from build123d import *

# Parameters (mm, degrees)
F1_W         = 50
F1_H         = 100
F2_DEPTH     = 30
F4_W         = 40
F4_H         = 90
F5_DEPTH     = 28
F6_SIZE      = 5
F7_T1_DEPTH  = 115
F7_T3_DEPTH  = 65
F8_W         = 40
F8_H         = 20
F9_DEPTH     = 40
F10_R        = 15.7450666382
F11_DEPTH    = 40
F12_R        = 5
F13_T1_DEPTH = 6.3508529611
F13_T3_DEPTH = 6.3508529611
F13_T5_DEPTH = 40.7168298797
F13_T7_DEPTH = 65.7168298797
F13_T9_DEPTH = 52.8584149398


# Not quite as in the source:
# - a fillet or chamfer that OpenCascade refuses, or shapes differently, is made with other operations: its cross-section is extruded or revolved along the edge and cut away or added


with BuildPart() as f2:
    # F1 (on face) → F2 (new body)
    with BuildSketch(Plane.XZ):
        Rectangle(F1_W, F1_H)
    extrude(amount=F2_DEPTH)

    # F4 (on face) → F5 (cut)
    with BuildSketch(Plane.XZ.offset(30)):
        with Locations((-0.4633623362, -0.2909506857)):
            Rectangle(F4_W, F4_H)
    extrude(amount=-F5_DEPTH, mode=Mode.SUBTRACT)

    # F6
    f6_edges = [f2.edges().sort_by_distance(p)[0] for p in [
        (25, -15, 50),
        (-25, -15, 50),
        (-25, -15, -50),
        (25, -15, -50),
    ]]
    chamfer(f6_edges, length=F6_SIZE)

    # F7: fillet of radius 5 on 4 edges, made by hand

    # F7_s2 → F7_t1 (cut)
    with BuildSketch(Plane.XY.offset(-57.5)):
        with BuildLine():
            ThreePointArc((-20, -30), (-23.5355339059, -28.5355339059), (-25, -25))
            Line((-25, -25), (-25, -30))
            Line((-25, -30), (-20, -30))
        make_face()
        with BuildLine():
            ThreePointArc((20, -30), (23.5355339059, -28.5355339059), (25, -25))
            Line((25, -25), (25, -30))
            Line((25, -30), (20, -30))
        make_face()
    extrude(amount=F7_T1_DEPTH, mode=Mode.SUBTRACT)

    # F7_s4 → F7_t3 (cut)
    with BuildSketch(Plane.YZ.offset(-32.5)):
        with BuildLine():
            ThreePointArc((-30, 45), (-28.5355339059, 48.5355339059), (-25, 50))
            Line((-25, 50), (-30, 50))
            Line((-30, 50), (-30, 45))
        make_face()
        with BuildLine():
            ThreePointArc((-25, -50), (-28.5355339059, -48.5355339059), (-30, -45))
            Line((-30, -45), (-30, -50))
            Line((-30, -50), (-25, -50))
        make_face()
    extrude(amount=F7_T3_DEPTH, mode=Mode.SUBTRACT)

    # F8 (on face) → F9 (join)
    with BuildSketch(Plane(origin=(0, 0, -50), x_dir=(1, 0, 0), z_dir=(0, 0, -1))):
        with Locations((0, 12.041676566)):
            Rectangle(F8_W, F8_H)
    extrude(amount=F9_DEPTH)

    # F10 (on face) → F11 (join)
    with BuildSketch(Plane.XZ.offset(22.041676566)):
        with Locations((0, -69.2195519805)):
            Circle(F10_R)
    extrude(amount=F11_DEPTH)

    # F12
    f12_edges = [f2.edges().sort_by_distance(p)[0] for p in [
        (-20, -22.041677, -70),
        (20, -22.041677, -70),
        (0, -22.041677, -90),
    ]]
    fillet(f12_edges, radius=F12_R)

    # F13: chamfer of 5 on 7 edges, made by hand

    # F13_s2 → F13_t1 (cut)
    with BuildSketch(Plane(origin=(-32.652774478, 32.652774478, -32.652774478), x_dir=(-0.7071067812, -0.7071067812, 0), z_dir=(-0.5773502692, 0.5773502692, -0.5773502692))):
        Polygon((12.0502850626, -64.1119959897), (19.1213528745, -64.1119959897), (15.5858189685, -70.2357203466), align=None)
    extrude(amount=F13_T1_DEPTH, mode=Mode.SUBTRACT)

    # F13_s4 → F13_t3 (cut)
    with BuildSketch(Plane(origin=(32.652774478, 32.652774478, -32.652774478), x_dir=(-0.7071067812, 0.7071067812, 0), z_dir=(0.5773502692, 0.5773502692, -0.5773502692))):
        Polygon((-19.1213528745, -64.1119959897), (-15.5858189685, -70.2357203466), (-12.0502850626, -64.1119959897), align=None)
    extrude(amount=F13_T3_DEPTH, mode=Mode.SUBTRACT)

    # F13_s6 → F13_t5 (cut)
    with BuildSketch(Plane.XZ.offset(-10.8167383738)):
        Polygon((-15, -90), (-20, -85), (-20, -90), align=None)
        Polygon((20, -85), (15, -90), (20, -90), align=None)
    extrude(amount=F13_T5_DEPTH, mode=Mode.SUBTRACT)

    # F13_s8 → F13_t7 (cut)
    with BuildSketch(Plane.YZ.offset(-32.8584149398)):
        Polygon((-2.041676566, -85), (-7.041676566, -90), (-2.041676566, -90), align=None)
    extrude(amount=F13_T7_DEPTH, mode=Mode.SUBTRACT)

    # F13_s10 → F13_t9 (cut)
    with BuildSketch(Plane.XY.offset(-102.8584149398)):
        Polygon((20, -7.041676566), (15, -2.041676566), (20, -2.041676566), align=None)
        Polygon((-15, -2.041676566), (-20, -7.041676566), (-20, -2.041676566), align=None)
    extrude(amount=F13_T9_DEPTH, mode=Mode.SUBTRACT)

    # F13_s11 → F13_t12 (revolve, cut)
    with BuildSketch(Plane.XY.offset(-69.2195519805)):
        Polygon((15.7450666382, -57.041676566), (10.7450666382, -62.041676566), (15.7450666382, -62.041676566), align=None)
    revolve(axis=Axis((0, -62.041676566, -69.2195519805), (0, -1, 0)), mode=Mode.SUBTRACT)


solid = f2.part
Model file for the job. Use its own axes, mm. A direction names the side the tool comes from. Round coordinates to 2 decimals unless told otherwise and drop trailing zeros. Loops run counter-clockwise (first coordinate to the right, second up) from the corner with the lowest first, then second, coordinate; pieces in that order, holes last. Notation, with made-up numbers: (-24, -35) -> (31, -35) arc R18 cw to (31, -13) -> close; hole circle Ø2 at (6, 64). An arc over 180 degrees is marked (long way). Answer as CSV lines item,"result". Start each with the question number.
1) Slice it at A-A (y = -15). List the corners of the cut face in (x, z).
2) Mould opens along Z. For faces 4 (the face through (-22, -14, -48)), 5 (the face through (-1, -16, -45.291)), 6 (the face through (20, -12, -67)) say: +Z half, -Z half, draft (parallel to the pull), parting line (faces both ways), or undercut.
3) Tool access for faces 1 (the face through (17.54, -4.58, -67.75)), 2 (the face through (-1, -16, 44.709)), 3 (the face through (18.57, -20.54, -57.32)): list every direction of +Z, -Z, +X, -X, +Y, -Y with a clear straight run to the whole face (end or side of a thin tool).
4) Slice it at B-B (z = -4). List the corners of the cut face in (x, y).
5) Slice it at D-D (y = -55). List the corners of the cut face in (x, z).
6) Probe line 1 along X through (y, z) = (-10.5, 31); line 2 along Z through (x, y) = (12, -23); line 3 along Z through (x, y) = (-1, -23.5). List the from-to ranges inside material, lowest first.
7) Pin check, flat tips, straight feed: P1, Ø12, axis at x = 2.5, z = -12.5, coming from the -Y side; P2, Ø5.5, axis at x = -5, y = -3, coming from the -Z side; P3, Ø5, axis at y = -13, z = -65.5, coming from the -X side. Stop position of each tip, or through.
Filled in:
1,outline,"(-25, -45) -> (-20, -50) -> (-20, -85) -> (-15, -90) -> (15, -90) -> (20, -85) -> (20, -50) -> (25, -45) -> (25, 45) -> (20, 50) -> (-20, 50) -> (-25, 45) -> close; hole (-20.46, -45.29) -> (19.54, -45.29) -> (19.54, 44.71) -> (-20.46, 44.71) -> close"
2,face 4,"-Z half"
2,face 5,"undercut"
2,face 6,"draft"
3,face 1,"-Z, +X, +Y"
3,face 2,"-Y"
3,face 3,"+X, -Y"
4,outline,"(-25, -25) arc R5 ccw to (-20.46, -29.98) -> (-20.46, -2) -> (19.54, -2) -> (19.54, -30) -> (20, -30) arc R5 ccw to (25, -25) -> (25, 0) -> (-25, 0) -> close"
5,outline,"circle Ø31.49 at (0, -69.22)"
6,line 1,"x = -25 to -20.46, 19.54 to 25"
6,line 2,"z = -79.41 to -59.03, -50 to -45.29, 44.71 to 50"
6,line 3,"z = -84.93 to -53.51, -50 to -45.29, 44.71 to 50"
7,P1,"stops at y = -2"
7,P2,"stops at z = -88.71"
7,P3,"stops at x = -20"
